Input: part model. Units: mm. Frame: model coordinates. A direction names the side the tool comes from. Coordinates: 2 decimals unless noted, no trailing zeros. Write each loop counter-clockwise with the first axis right and the second up, starting at its lowest first coordinate (ties: lowest second). Pieces come first, ordered by that corner, then holes. Notation, with made-up numbers: M 36.25,85 L 57.25,85 A16 ccw 57.25,104 Z; hole C 5,-28.75 d10. An arc over 180 degrees is marked long. Use one line per item in the form item = value.
Autodesk Inventor part; units mm, degrees
ref_plane "YZ Plane" through (0, 0, 0) normal (1, 0, 0) x (0, 1, 0)
ref_plane "XZ Plane" through (0, 0, 0) normal (0, 1, 0) x (-1, 0, 0)
ref_plane "XY Plane" through (0, 0, 0) normal (0, 0, 1) x (1, 0, 0)
sketch "Sketch1" plane through (0, 0, 0) normal (0, 0, 1) x (1, 0, 0)
  line L0 (10, -206) -> (-10, -206) construction
  line L1 (0, 0) -> (0, -45.7411)
  line L2 (-10, -206) -> (10, -206) construction
  arc A0 (-10, -160.3333) -> (10, -160.3333) centre (0, -160.3333) ccw
  line L3 (10, -143.6667) -> (10, -160.3333)
  line L4 (-10, -160.3333) -> (-10, -143.6667)
  arc A1 (10, -143.6667) -> (-10, -143.6667) centre (0, -143.6667) ccw
  circle A2 centre (-8, -187) radius 1.6
  circle A3 centre (8, -187) radius 1.6
  arc A4 (-5.8349, -87.227) -> (5.8349, -87.227) centre (0, -87.227) ccw
  line L5 (5.8349, -53.3669) -> (5.8349, -87.227)
  line L6 (-5.8349, -87.227) -> (-5.8349, -53.3669)
  arc A5 (5.8349, -53.3669) -> (-5.8349, -53.3669) centre (0, -53.3669) ccw
  line L7 (0, -206) -> (-90.9613, -206)
  line L8 (-90.9613, -206) -> (-90.9613, -180.2754)
  arc A6 (-90.9613, -180.2754) -> (-22, -103.3247) centre (-99.4135, -103.3247) ccw
  line L9 (-22, -103.3247) -> (-22, 74.3972)
  line L10 (0, -143.6667) -> (0, -187) construction
  line L11 (-13, -143.6667) -> (-13, -187)
  line L12 (13, -187) -> (13, -143.6667)
  arc A7 (13, -143.6667) -> (-13, -143.6667) centre (0, -143.6667) ccw
  arc A8 (-13, -187) -> (13, -187) centre (0, -187) ccw
  line L13 (0, -206) -> (90.9613, -206)
  line L14 (90.9613, -206) -> (90.9613, -180.2754)
  arc A9 (22, -103.3247) -> (90.9613, -180.2754) centre (99.4135, -103.3247) ccw
  line L15 (22, -103.3247) -> (22, 74.3972)
  line L16 (5.8349, 46.6331) -> (5.8349, 12.773)
  arc A10 (-5.8349, 12.773) -> (5.8349, 12.773) centre (0, 12.773) ccw
  line L17 (-5.8349, 12.773) -> (-5.8349, 46.6331)
  arc A11 (5.8349, 46.6331) -> (-5.8349, 46.6331) centre (0, 46.6331) ccw
  line L18 (-22, 74.3972) -> (22, 74.3972)
  point P0 (0, -165.3333)
  dimension "d2" = 26
  dimension "d5" = 22
extrude "Extrusion1" add sketch "Sketch1" along normal blind 6 contours L7 L8 A6 L9 L18 L15 A9 L14 L13
properties part number "Camera stabiliser"
(1) Section query A-A on y = -73.5. Return the cut outline in (x, z), plus the area to 3 significant figures.
Computed:
outline = M -22,0 L -5.83,0 L -5.83,6 L -22,6 Z; M 5.83,0 L 22,0 L 22,6 L 5.83,6 Z
area = 194 mm^2
(2) First-contact query: pin 1 Ø1 at (x, z) = (-57.5, 3) entering from +Y; pin 2 Ø1.8 at (y, z) = (34.5, 1.5) entering from -X; pin 3 Ø2 at (x, y) = (-11, 7) entering from -Z; pin 4 Ø1.8 at (y, z) = (-13.5, 3) entering from +X. Flat tips, straight axial feed; report the tip coordinate or a pass-through.
Computed:
pin_1 = -168.09
pin_2 = -22
pin_3 = 0
pin_4 = 22
(3) Section query D-D on y = -44. Return the cut outline in (x, z).
Computed:
outline = M -22,0 L 22,0 L 22,6 L -22,6 Z
(4) Pull-direction query (Y, two-part tool) for faces 1 (the cylindrical face through (-0.128, 52.467, 2.958)), 2 (the flat face through (-1, -206, 3)), 3 (the flat face through (-1, -95, 0)); classes: pulls with the +Y half, pulls with the -Y half, needs draft (parallel to the pull), parting line crosses it, or undercut.
Computed:
face_1 = undercut
face_2 = pulls with the -Y half
face_3 = needs draft
(5) Section query C-C on z = 3.75. Return the cut outline in (x, y), plus the area to 3 significant figures.
Computed:
outline = M -90.96,-206 L 90.96,-206 L 90.96,-180.28 A77.41 cw 22,-103.32 L 22,74.4 L -22,74.4 L -22,-103.32 A77.41 cw -90.96,-180.28 Z; hole M -13,-187 A13 ccw 13,-187 L 13,-143.67 A13 ccw -13,-143.67 Z; hole M -5.83,-87.23 A5.83 ccw 5.83,-87.23 L 5.83,-53.37 A5.83 ccw -5.83,-53.37 Z; hole M -5.83,12.77 A5.83 ccw 5.83,12.77 L 5.83,46.63 A5.83 ccw -5.83,46.63 Z
area = 15,700 mm^2
(6) Section query B-B on x = 0. Return the cut outline in (y, z), plus the area to 3 significant figures.
Computed:
outline = M -206,0 L -200,0 L -200,6 L -206,6 Z; M -130.67,0 L -93.06,0 L -93.06,6 L -130.67,6 Z; M -47.53,0 L 6.94,0 L 6.94,6 L -47.53,6 Z; M 52.47,0 L 74.4,0 L 74.4,6 L 52.47,6 Z
area = 720 mm^2
(7) Set-up query: faces 4 (the flat face through (-22, -16, 3)), 5 (the flat face through (-1, -95, 6)), 6 (the flat face through (-5.835, -71, 3)). Return all of +Z, -Z, +X, -X, +Y, -Y with unobstructed straight access to the full face (end or side cutting, diameter ignored); none if empty.
Computed:
face_4 = +Z, -Z, -X, +Y
face_5 = +Z, +X, -X, +Y, -Y
face_6 = +Z, -Z
(8) Line query: probe 1 along X at (y, z) = (16, 3.8); probe 2 along X at (y, z) = (-186.5, 2.15); probe 3 along X at (y, z) = (-12.5, 5.15). Output: solid intervals per line, ascending.
Computed:
probe_1 = -22 to -5.83, 5.83 to 22
probe_2 = -90.96 to -13, 13 to 90.96
probe_3 = -22 to 22
